Verification items for the finished model (mm, model axes). Face numbers are marked on the shaded views. A direction names the side the tool comes from. Coordinates: 2 decimals unless noted, no trailing zeros. Order: outer loops, then holes, each group sorted by start corner. A loop starts at its lowest first (then second) coordinate and runs counter-clockwise, first axis right, second up. Notation, with made-up numbers: M -12.5,26 L 28.5,26 A28 cw 28.5,52 Z; hole C -0.75,-1.75 d4. An arc over 180 degrees is marked long. Return JSON: item names as keys, results as strings.
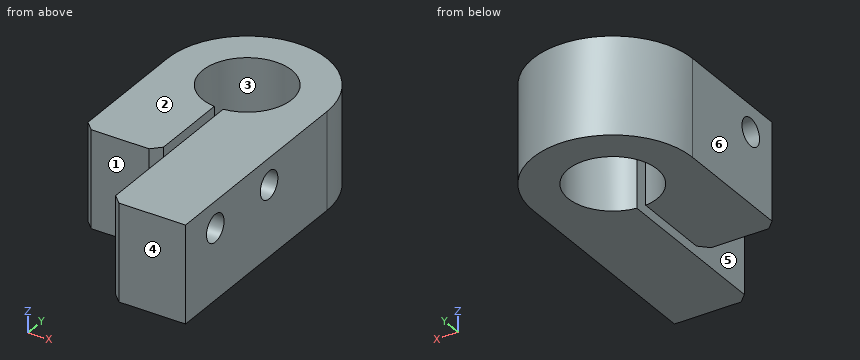
Autodesk Inventor part; units mm, degrees
ref_plane "YZ Plane" through (0, 0, 0) normal (1, 0, 0) x (0, 1, 0)
ref_plane "XZ Plane" through (0, 0, 0) normal (0, 1, 0) x (-1, 0, 0)
ref_plane "XY Plane" through (0, 0, 0) normal (0, 0, 1) x (1, 0, 0)
sketch "Szkic1" plane through (0, 0, 0) normal (0, 0, 1) x (1, 0, 0)
  arc A0 (0.5, -5.0252) -> (-0.5, -5.0252) centre (0, 0) ccw
  arc A1 (0.5, -9.0362) -> (-0.5, -9.0362) centre (0, 0) ccw
  line L0 (-9.05, 0) -> (-9.05, -25)
  line L1 (-9.05, -25) -> (-0.5, -25)
  line L2 (9.05, 0) -> (9.05, -25)
  line L3 (9.05, -25) -> (0.5, -25)
  line L4 (-0.5, -25) -> (-0.5, -5.0252)
  line L5 (0.5, -25) -> (0.5, -5.0252)
  dimension "d0" = 10.1
  dimension "d1" = 4
  dimension "d2" = 8.55
  dimension "d3" = 8.55
  dimension "d4" = 25
  dimension "d5" = 25
  dimension "d7" = 1
extrude "Wyciągnięcie proste1" add sketch "Szkic1" along normal blind 11
sketch "Szkic2" plane through (9.05, -25, 0) normal (1, 0, 0) x (0, 0, -1)
  line L0 (0, 0) -> (0, 25)
  line L1 (0, 25) -> (-11, 25)
  line L2 (-11, 0) -> (-11, 25)
  line L3 (0, 0) -> (-11, 0)
  line L4 (0, 20) -> (-11, 20)
  line L5 (-11, 25) -> (-11, 0)
  point P0 (-8, 5.25)
  point P1 (-8, 14.75)
  dimension "d10" = 5.25
  dimension "d11" = 20
  dimension "d12" = 5.25
  dimension "d13" = 11
  dimension "d14" = 3
  dimension "d15" = 3
hole "Otwór1" at (9.05, -19.75, 8) at (9.05, -10.25, 8) direction (-1, 0, 0) diameter 3.1 end through all
sketch "Szkic3" plane through (-9.05, -25, 0) normal (0, -1, 0) x (1, 0, 0)
  line L0 (0, 0) -> (8.55, 0)
  line L1 (8.55, 0) -> (8.55, 11)
  line L2 (0, 11) -> (8.55, 11)
  line L3 (0, 0) -> (0, 11)
  point P0 (9.05, 0)
extrude "Wyciągnięcie proste2" cut sketch "Szkic3" against normal blind 10
chamfer "Faza1" distance 1 angle 45 3 edges at (-9.05, -15, 5.5) (-0.5, -15, 5.5) (0.5, -25, 5.5)
equation "\"d3\" = d2"
equation "\"d4\" = d5"
properties part number "3DP_ABS_X_Axis_Endstop_Mount"
Q1. Draft check along X on the marked faces 3, 4, 5 and 6. Enter one of: pulls with the +X half, pulls with the -X half, needs draft (parallel to the pull), parting line crosses it, or undercut.
Values:
{"face 3": "undercut", "face 4": "needs draft", "face 5": "undercut", "face 6": "pulls with the -X half"}
Q2. Cross-section at B-B, the plane z = 8. Record the boundary of the cut face in (x, y).
Values:
{"outline": "M -9.05,-14 L -8.05,-15 L -1.5,-15 L -0.5,-14 L -0.5,-11.8 L -9.05,-11.8 Z; M -9.05,-8.7 L -0.5,-8.7 L -0.5,-5.03 A5.05 cw long 0.5,-5.03 L 0.5,-8.7 L 9.05,-8.7 L 9.05,0 A9.05 ccw -9.05,0 Z; M 0.5,-24 L 1.5,-25 L 9.05,-25 L 9.05,-21.3 L 0.5,-21.3 Z; M 0.5,-18.2 L 9.05,-18.2 L 9.05,-11.8 L 0.5,-11.8 Z"}
Q3. Cross-section at A-A, the plane y = -10.25. Record the boundary of the cut face in (x, z).
Values:
{"outline": "M -9.05,0 L -0.5,0 L -0.5,6.45 L -9.05,6.45 Z; M -9.05,9.55 L -0.5,9.55 L -0.5,11 L -9.05,11 Z; M 0.5,0 L 9.05,0 L 9.05,6.45 L 0.5,6.45 Z; M 0.5,9.55 L 9.05,9.55 L 9.05,11 L 0.5,11 Z"}
Q4. Tool access check on the marked faces 1 and 2. Record the directions out of +Z, -Z, +X, -X, +Y, -Y that give a thin tool (end or side, any length) a straight path to the whole face; none if there is none.
Values:
{"face 1": "+Z, -Z, -X, -Y", "face 2": "+Z, +X, -X, +Y, -Y"}
Q5. Go/stop test with flat-tipped pins: pin 1 (5 mm diameter, centred on x = 6.5, z = 1.5, fed in from +Y); pin 2 (2 mm diameter, centred on y = 5, z = 1.5, fed in from -X); pin 3 (5 mm diameter, centred on x = -6, z = 7.5, fed in from -Y). Record where each tip stops, or that it passes through.
Values:
{"pin 1": "y = 8.12", "pin 2": "x = -8.12", "pin 3": "y = -15"}
Q6. Material ranges on line 1 along Z through (x, y) = (-4.75, -10.25); line 2 along Y through (x, z) = (5.5, 8.5); line 3 along X through (y, z) = (-5.5, 2), recorded low to high.
Values:
{"line 1": "0 to 6.45, 9.55 to 11", "line 2": "-25 to -21.22, -18.28 to -11.72, -8.78 to 7.19", "line 3": "-9.05 to -0.5, 0.5 to 9.05"}
Q7. Cross-section at C-C, the plane y = -19.75. Record the boundary of the cut face in (x, z), and give its area (3 significant figures).
Values:
{"outline": "M 0.5,0 L 9.05,0 L 9.05,6.45 L 0.5,6.45 Z; M 0.5,9.55 L 9.05,9.55 L 9.05,11 L 0.5,11 Z", "area": "67.5 mm^2"}
Q8. Cross-section at D-D, the plane z = 3. Record the boundary of the cut face in (x, y), and give its area (3 significant figures).
Values:
{"outline": "M -9.05,-14 L -8.05,-15 L -1.5,-15 L -0.5,-14 L -0.5,-5.03 A5.05 cw long 0.5,-5.03 L 0.5,-24 L 1.5,-25 L 9.05,-25 L 9.05,0 A9.05 ccw -9.05,0 Z", "area": "394 mm^2"}
